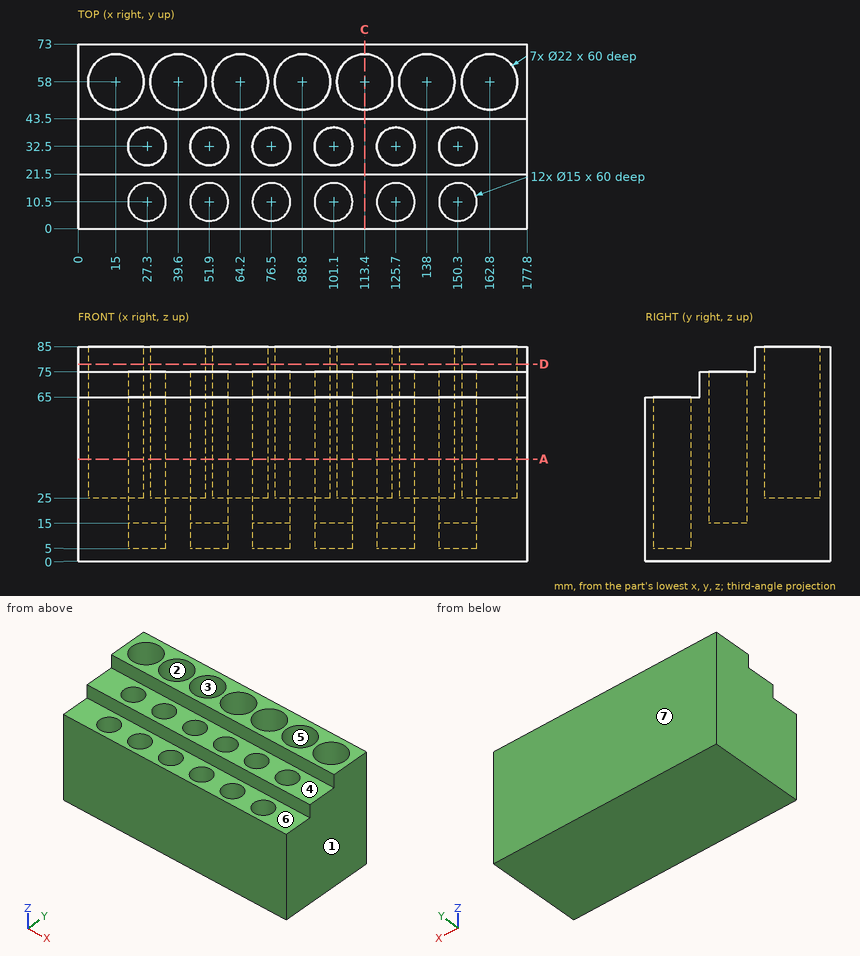
Can you work these out from the drawing? Everything is in mm from the part's minimum corner. A direction names the side the tool comes from. Give positions to 0.01 mm unless a question says otherwise; leave off trailing zeros. Loops run counter-clockwise (first coordinate to the right, second up) from the corner with the lowest first, then second, coordinate; pieces in that order, holes last. Notation, with made-up numbers: M -18,20 L 22,20 A17 ccw 22,30 Z; hole C 89,-36 d7. An arc over 180 degrees is marked long. Put each result on its own line as item: value. Start each with the question number.
(1) I need wall thicknesses on line 1 along Y through (x, z) = (76.5, 37); line 2 along Y through (x, z) = (113.4, 40.5); line 3 along Y through (x, z) = (148, 18). Which ranges of each line are inside material? Lowest first, please. Write a range as [from, to].
(2) If we mould it in two halves opening along X, with no side actions, what happens to the marked faces 1, 2, 3 and 4? For each: +X half, -X half, draft (parallel to the pull), parting line (faces both ways), or undercut.
(3) For the marked faces 5, 6 and 7, which set-ups out of +Z, -Z, +X, -X, +Y, -Y let a thin tool reach every point of the face, with its end or its side?
(4) I want a section at D-D on z = 78. Please give me the cut outline in (x, y).
(5) I want a section at A-A on z = 40.5. State how many separate pieces and enclosed holes the cut face has, then the cut area to 3 significant figures.
(6) Will these pins go through, and if not, where does the flat tip stop? pin 1 Ø12 at (x, y) = (74.5, 29) entering from +Z; pin 2 Ø16.5 at (x, y) = (75, 11.5) entering from +Z; pin 3 Ø4.5 at (x, y) = (129.5, 32) entering from +Z.
(7) I want a section at C-C on x = 113.4. Please give me the cut outline in (y, z).
Answer block:
1. line 1: [0, 3], [18, 25], [40, 73]
1. line 2: [0, 47], [69, 73]
1. line 3: [0, 3.36], [17.64, 25.36], [39.64, 73]
2. face 1: +X half
2. face 2: undercut
2. face 3: undercut
2. face 4: draft
3. face 5: +Z
3. face 6: +Z, +X, -X, -Y
3. face 7: +Z, -Z, +X, -X, +Y
4. outline: M 0,43.5 L 177.8,43.5 L 177.8,73 L 0,73 Z; hole C 15,58 d22; hole C 39.6,58 d22; hole C 64.2,58 d22; hole C 88.8,58 d22; hole C 113.4,58 d22; hole C 138,58 d22; hole C 162.8,58 d22
5. separate pieces: 1
5. enclosed holes: 19
5. area: 8,200 mm^2
6. pin 1: z = 75
6. pin 2: z = 65
6. pin 3: z = 15
7. outline: M 0,0 L 73,0 L 73,85 L 69,85 L 69,25 L 47,25 L 47,85 L 43.5,85 L 43.5,75 L 21.5,75 L 21.5,65 L 0,65 Z
